Source: CAD feature listing. Evaluate the final solid. Frame: model axes, mm. A direction names the side the tool comes from. Round coordinates to 2 decimals unless told otherwise and drop trailing zeros. Write each loop counter-clockwise with the first axis right and the second up, starting at its lowest first coordinate (ties: lowest second). Pieces come first, ordered by that corner, then holes.
Autodesk Inventor part; units mm, degrees
ref_plane "YZ Plane" through (0, 0, 0) normal (1, 0, 0) x (0, 1, 0)
ref_plane "XZ Plane" through (0, 0, 0) normal (0, 1, 0) x (-1, 0, 0)
ref_plane "XY Plane" through (0, 0, 0) normal (0, 0, 1) x (1, 0, 0)
sketch "Sketch1" plane through (0, 0, 0) normal (0, 1, 0) x (-1, 0, 0)
  line L0 (-13, -31) -> (13, -31)
  line L1 (13, -31) -> (13, 31)
  line L2 (13, 31) -> (-13, 31)
  line L3 (-13, 31) -> (-13, -31)
  line L4 (-13, -31) -> (13, 31) construction
  line L5 (13, -31) -> (-13, 31) construction
  point P0 (0, 0)
  dimension "d0" = 26
  dimension "d1" = 62
extrude "Extrusion1" add sketch "Sketch1" along normal blind 1.3
sketch "Sketch2" plane through (0, 1.3, 0) normal (0, 1, 0) x (1, 0, 0)
  line L0 (-8, 26) -> (0, 26)
  line L1 (0, 26) -> (0, 32)
  line L2 (0, 32) -> (-8, 32)
  line L3 (-8, 32) -> (-8, 26)
  line L4 (13, 31) -> (-13, 31)
  line L5 (-13, 31) -> (-13, -31)
  point P0 (0, 0)
  dimension "d4" = 8
  dimension "d5" = 6
  dimension "d6" = 1
  dimension "d7" = 5
extrude "Extrusion2" add sketch "Sketch2" along normal blind 3
sketch "Sketch3" plane through (-13, 0, -31) normal (-1, 0, 0) x (0, 0, 1)
  line L0 (16.6, 2.6) -> (5.6, 2.6)
  line L1 (5.6, 2.6) -> (5.6, 4.1)
  line L2 (5.6, 4.1) -> (16.6, 4.1)
  line L3 (16.6, 4.1) -> (16.6, 2.6)
  line L4 (0, 0) -> (62, 0)
  line L5 (0, 0) -> (0, 1.3)
  point P0 (31, 0)
  dimension "d10" = 11
  dimension "d11" = 1.5
  dimension "d12" = 2.6
  dimension "d13" = 5.6
extrude "Extrusion3" add sketch "Sketch3" along normal blind 9.2 and the other way blind 5.8
sketch "Sketch4" plane through (0, 1.3, 0) normal (0, 1, 0) x (1, 0, 0)
  line L0 (-13, 31) -> (-13, -31)
  line L1 (-7.2, 25.4) -> (-22.2, 25.4)
  line L2 (-7.2, 14.4) -> (-22.2, 14.4)
  line L3 (-7.2, 25.4) -> (-13, 25.4)
  line L4 (-13, 25.4) -> (-13, 14.4)
  line L5 (-13, 14.4) -> (-7.2, 14.4)
  line L6 (-7.2, 14.4) -> (-7.2, 25.4)
  point P0 (0, 0)
  point P1 (-13, 25.4)
extrude "Extrusion4" add sketch "Sketch4" along normal up to surface (2.8 mm away)
sketch "Sketch5" plane through (13, 0, 31) normal (1, 0, 0) x (0, 0, -1)
  line L0 (46, 3.3) -> (53, 3.3)
  line L1 (53, 3.3) -> (53, 1.3)
  line L2 (53, 1.3) -> (46, 1.3)
  line L3 (46, 1.3) -> (46, 3.3)
  line L4 (0, 1.3) -> (62, 1.3)
  line L5 (62, 0) -> (62, 1.3)
  point P0 (31, 0)
  dimension "d20" = 16
  dimension "d21" = 7
  dimension "d22" = 2
extrude "Extrusion5" add sketch "Sketch5" against normal blind 3
sketch "Sketch6" plane through (13, 0, 31) normal (1, 0, 0) x (0, 0, -1)
  line L0 (48, 2.5) -> (49.2, 2.5)
  line L1 (49.2, 2.5) -> (49.2, 1.5)
  line L2 (49.2, 1.5) -> (48, 1.5)
  line L3 (48, 1.5) -> (48, 2.5)
  line L4 (62, 0) -> (62, 1.3)
  line L5 (0, 0) -> (62, 0)
  point P0 (31, 0)
  dimension "d25" = 1.2
  dimension "d26" = 1
  dimension "d27" = 14
  dimension "d28" = 2.5
extrude "Extrusion6" add sketch "Sketch6" along normal blind 0.5
pattern_linear "Rectangular Pattern1" count 2 spacing 1.5 along (0, 0, -1) of "Extrusion6"
sketch "Sketch7" plane through (0, 1.3, -32) normal (0, 0, -1) x (-1, 0, 0)
  line L0 (0, 0) -> (8, 0)
  line L1 (8, 0) -> (8, 3)
  line L2 (0, 3) -> (8, 3)
  line L3 (0, 0) -> (0, 3)
  line L4 (7.5, 2.5) -> (7.5, 0.5)
  line L5 (7.5, 0.5) -> (0.5, 0.5)
  line L6 (0.5, 0.5) -> (0.5, 2.5)
  line L7 (0.5, 2.5) -> (7.5, 2.5)
  point P0 (0, -1.3)
  dimension "d34" = 0.5
extrude "Extrusion7" add sketch "Sketch7" along normal blind 0.5 contours L4 L5 L6 L7
sketch "Sketch8" plane through (0, 1.3, -32.5) normal (0, 0, -1) x (-1, 0, 0)
  line L0 (7.5, 2.5) -> (0.5, 2.5)
  line L1 (0.5, 2.5) -> (0.5, 0.5)
  line L2 (0.5, 0.5) -> (7.5, 0.5)
  line L3 (7.5, 0.5) -> (7.5, 2.5)
  line L4 (9, 5) -> (-1, 5)
  line L5 (-1, 5) -> (-1, -2)
  line L6 (-1, -2) -> (9, -2)
  line L7 (9, -2) -> (9, 5)
  line L8 (9, 5) -> (-1, -2) construction
  line L9 (-1, 5) -> (9, -2) construction
  point P0 (0, -1.3)
  point P1 (4, 1.5)
  dimension "d37" = 10
  dimension "d38" = 7
extrude "Extrusion8" add sketch "Sketch8" along normal blind 10 contours L3 L2 L1 L0 | L7 L6 L5 L4
sketch "Sketch9" plane through (0, 1.3, 0) normal (0, 1, 0) x (1, 0, 0)
  line L0 (-13, -31) -> (13, -31)
  line L1 (-8.5, -31) -> (6.5, -31)
  line L2 (6.5, -31) -> (6.5, -25.5)
  line L3 (6.5, -25.5) -> (-8.5, -25.5)
  line L4 (-8.5, -25.5) -> (-8.5, -31)
  line L5 (-13, 14.4) -> (-13, -31)
  point P0 (0, 0)
  dimension "d41" = 15
  dimension "d42" = 5.5
  dimension "d43" = 4.5
extrude "Extrusion9" add sketch "Sketch9" along normal blind 5
sketch "Sketch10" plane through (0, 1.3, 0) normal (0, 1, 0) x (1, 0, 0)
  line L0 (-8.5, -10.5) -> (-7.1, -10.5)
  line L1 (-7.1, -10.5) -> (-7.1, -9.7)
  line L2 (-7.1, -9.7) -> (-8.5, -9.7)
  line L3 (-8.5, -9.7) -> (-8.5, -10.5)
  line L4 (-13, 14.4) -> (-13, -31)
  line L5 (-13, -31) -> (-8.5, -31)
  line L6 (5.5, 15) -> (4.1, 15)
  line L7 (4.1, 15) -> (4.1, 14.2)
  line L8 (4.1, 14.2) -> (5.5, 14.2)
  line L9 (5.5, 14.2) -> (5.5, 15)
  line L10 (13, -31) -> (13, 15)
  line L11 (13, 31) -> (0, 31)
  point P0 (0, 0)
  dimension "d46" = 4.5
  dimension "d47" = 20.5
  dimension "d48" = 0.8
  dimension "d49" = 1.4
  dimension "d50" = 7.5
  dimension "d51" = 16
  dimension "d52" = 0.8
  dimension "d53" = 1.4
extrude "Extrusion10" add sketch "Sketch10" along normal blind 20
sketch "Sketch11" plane through (13, 0, 31) normal (1, 0, 0) x (0, 0, -1)
  line L0 (49.5, 2.5) -> (50.7, 2.5)
  line L1 (50.7, 2.5) -> (50.7, 1.5)
  line L2 (50.7, 1.5) -> (49.5, 1.5)
  line L3 (49.5, 1.5) -> (49.5, 2.5)
  line L4 (48, 2.5) -> (49.2, 2.5)
  line L5 (49.2, 2.5) -> (49.2, 1.5)
  line L6 (49.2, 1.5) -> (48, 1.5)
  line L7 (48, 1.5) -> (48, 2.5)
  line L8 (0, 0) -> (62, 0)
  line L9 (62, 0) -> (62, 1.3)
  line L10 (53, 1.3) -> (62, 1.3)
  line L11 (53, 1.3) -> (53, 3.3)
  line L12 (53, 3.3) -> (46, 3.3)
  line L13 (46, 3.3) -> (46, 1.3)
  line L14 (0, 1.3) -> (46, 1.3)
  line L15 (0, 0) -> (0, 1.3)
  line L16 (46, 1.3) -> (53, 1.3)
  line L17 (46, 1.3) -> (53, 1.3)
  point P0 (31, 0)
extrude "Extrusion11" cut sketch "Sketch11" against normal blind 0.2 contours L13 L12 L11 L16
equation "\"d52\" = d48"
equation "\"d53\" = d49"
properties part number "esp32_t8"
1) Pull-direction query (Z, two-part tool) for faces 6 (the face through (0, 2, 31)), 7 (the face through (13, 1, 0)), 8 (the face through (-8, 11, 9.7)); classes: released by +Z, released by -Z, zero draft, split by the parting line, or undercut.
Taken from the geometry:
face 6: released by +Z
face 7: zero draft
face 8: undercut
2) Section query C-C on z = 2.5. Return the cut outline in (x, y), then the cut area to 3 significant figures.
Taken from the geometry:
outline: (-13, 0) - (13, 0) - (13, 1.3) - (-13, 1.3) - close
area: 33.8 mm2
3) Contact query for flat-ended pins moving along their axis: P1, Ø4.5, axis at x = -1, z = 28.5, coming from the +Y side; P2, Ø2, axis at y = 6.5, z = -20, coming from the +X side; P3, Ø4, axis at x = -5, z = 14.5, coming from the -Y side; P4, Ø0.8, axis at x = 13.5, y = 2, coming from the -Z side. Output: stop coordinate, or through.
Taken from the geometry:
P1: stops at y = 6.3
P2: passes through
P3: stops at y = 0
P4: stops at z = -19.7
4) Section query D-D on x = 3. Return the cut outline in (y, z), then the cut area to 3 significant figures.
Taken from the geometry:
outline: (0, -31) - (1.3, -31) - (1.3, 25.5) - (6.3, 25.5) - (6.3, 31) - (0, 31) - close
area: 108 mm2
5) Reachability of faces 1 (the face through (11, 3.3, -18)), 2 (the face through (-9, 3, -37)), 3 (the face through (-8.5, 4, 28)), 4 (the face through (-13, 1, 0)), 5 (the face through (-4, 4.3, -29)) from +Z, -Z, +X, -X, +Y, -Y: full face, straight path, thin tool, end or side. Return the list, or none.
Taken from the geometry:
face 1: +Z, -Z, +X, +Y
face 2: -Z, -X, +Y, -Y
face 3: +Z, -X, +Y
face 4: +Z, -Z, -X, -Y
face 5: +X, -X, +Y
6) Section query B-B on x = -5.5. Return the cut outline in (y, z).
Taken from the geometry:
outline: (-0.7, -42.5) - (6.3, -42.5) - (6.3, -32.5) - (3.8, -32.5) - (3.8, -32) - (4.3, -32) - (4.3, -26) - (1.3, -26) - (1.3, 25.5) - (6.3, 25.5) - (6.3, 31) - (0, 31) - (0, -31) - (1.3, -31) - (1.3, -32) - (1.8, -32) - (1.8, -32.5) - (-0.7, -32.5) - close
7) Section query A-A on y = 11.5. Return the cut outline in (x, z).
Taken from the geometry:
outline: (-8.5, 9.7) - (-7.1, 9.7) - (-7.1, 10.5) - (-8.5, 10.5) - close; (4.1, -15) - (5.5, -15) - (5.5, -14.2) - (4.1, -14.2) - close
8) Material intervals for line 1 (Y direction, x = -9, z = -5.5); line 2 (Z direction, x = 12.5, y = 3); line 3 (X direction, y = 19.75, z = 10), sorted ascending.
Taken from the geometry:
line 1: y = 0 to 1.3
line 2: z = -22 to -15
line 3: x = -8.5 to -7.1
